Autodesk Inventor part; units mm, degrees
ref_plane "YZ Plane" through (0, 0, 0) normal (1, 0, 0) x (0, 1, 0)
ref_plane "XZ Plane" through (0, 0, 0) normal (0, 1, 0) x (-1, 0, 0)
ref_plane "XY Plane" through (0, 0, 0) normal (0, 0, 1) x (1, 0, 0)
sketch "Sketch1" plane through (0, 0, 0) normal (0, 0, 1) x (1, 0, 0)
  arc A0 (-6.0433, 18.066) -> (6.0433, -18.066) centre (0, 0) ccw
  arc A1 (84.3294, 8.1215) -> (72.2428, 44.2536) centre (78.2861, 26.1876) ccw
  line L0 (-6.0433, 18.066) -> (72.2428, 44.2536)
  line L1 (84.3294, 8.1215) -> (6.0433, -18.066)
  arc A2 (-7.5541, 22.5825) -> (7.5541, -22.5825) centre (0, 0) ccw
  arc A3 (85.8402, 3.605) -> (70.732, 48.7701) centre (78.2861, 26.1876) ccw
  line L2 (7.5541, -22.5825) -> (85.8402, 3.605)
  line L3 (70.732, 48.7701) -> (-7.5541, 22.5825)
  dimension "d0" = 19.05
  dimension "d1" = 82.55
  dimension "d2" = 4.7625
extrude "Extrusion1" add sketch "Sketch1" along normal blind 4.7625
fillet "Fillet1" radius 2.3813 8 edges at (-22.5825, -7.5541, 0) (46.6972, -9.4887, 0) (100.8686, 33.7417, 0) (31.5889, 35.6763, 0) (100.8686, 33.7417, 4.7625) (46.6972, -9.4887, 4.7625) (-22.5825, -7.5541, 4.7625) (31.5889, 35.6763, 4.7625)
properties part number "Belt_HorizontalIntake_Front" material "High Density Polyethylene"
Could you check a few things on this model? Use its own coordinates, in mm. A direction names the side the tool comes from. Give positions to 0.01 mm unless a question says otherwise; leave off trailing zeros. Order: outer loops, then holes, each group sorted by start corner. A loop starts at its lowest first (then second) coordinate and runs counter-clockwise, first axis right, second up. Notation, with made-up numbers: (85.25, -15) -> (140.25, -15) arc R21 ccw to (140.25, -7) -> close; hole circle Ø1 at (88, 0.25). An arc over 180 degrees is marked (long way). Answer in a Markdown table with one row per item. Add a question column.
Item 1: Imagine slicing it at A-A (z = 1.1). List the corners of the cut face in (x, y) for me, and give its area (3 significant figures).
Item 2: Please list where these lines run through material, in increasing order: probe 1 along Y at (x, z) = (-4.5, 3.7); probe 2 along Y at (x, z) = (64, 1.5); probe 3 along X at (y, z) = (14.5, 1.6).
Item 3: We'd pull the mould along Y, two halves only. Please class faces 3 (the cylindrical face through (47.03, -8.661, 0.716)), 4 (the cylindrical face through (96.215, 32.627, 2.348)), 5 (the flat face through (48, -5, 0)), 6 (the cylindrical face through (31.256, 34.849, 0.716)): pulls with the +Y half, pulls with the -Y half, needs draft (parallel to the pull), parting line crosses it, or undercut.
Item 4: For faces 1 (the cylindrical face through (31.268, 34.814, 4.083)), 2 (the flat face through (45.7, -4.8, 2.3)), which set-ups out of +Z, -Z, +X, -X, +Y, -Y let a thin tool reach every point of the face, with its end or its side?
Item 5: I'm going to push a flat-ended pin straight in: P1, Ø2, axis at y = 9.5, z = 1, coming from the -X side. Where does the tip first touch, or does it pass through?
Result:
| question | item | result |
|---|---|---|
| 1 | outline | (-7.44, 22.23) arc R23.44 ccw to (7.44, -22.23) -> (85.72, 3.96) arc R23.44 ccw to (70.85, 48.42) -> close; hole (-6.04, 18.07) arc R19.05 ccw to (6.04, -18.07) -> (84.33, 8.12) arc R19.05 ccw to (72.24, 44.25) -> close |
| 1 | area | 1,310 mm2 |
| 2 | probe 1 | -22.98 to -18.51, 18.58 to 23.18 |
| 2 | probe 2 | -3.52 to 1.32, 41.5 to 46.34 |
| 2 | probe 3 | -18.72 to -12.36, 93.33 to 98.88 |
| 3 | face 3 | pulls with the -Y half |
| 3 | face 4 | undercut |
| 3 | face 5 | needs draft |
| 3 | face 6 | pulls with the +Y half |
| 4 | face 1 | +Z, -X, +Y |
| 4 | face 2 | +Z, -Z |
| 5 | P1 | x = -22.03 |
